For this review, take the finished solid that the model builds, in its own axes (mm). A direction names the side the tool comes from. Coordinates: 2 decimals unless noted, no trailing zeros. Loops run counter-clockwise (first coordinate to the right, second up) from the corner with the lowest first, then second, coordinate; pieces in that order, holes last. Notation, with made-up numbers: (-39.75, 5) -> (7.25, 5) arc R5 ccw to (7.25, 10) -> close; hole circle Ø3 at (79.5, -27.5). An arc over 180 degrees is marked (long way). Answer in a Markdown table with one row per item.
from build123d import *

# Parameters (mm, degrees)
BOSS_EXTRUDE1_DEPTH                           = 1
BOSS_EXTRUDE2_DEPTH                           = 1.44
CUT_EXTRUDE1_DEPTH                            = 32.926898982
SKETCH4_W                                     = 11.303
SKETCH4_H                                     = 6.1214
CUT_EXTRUDE2_DEPTH                            = 0.551
CUT_EXTRUDE2_DRAFT                            = -45
SKETCH5_R                                     = 1.7907
BOSS_EXTRUDE3_DEPTH                           = 3.8354
CSK_FOR_4_FLAT_HEAD_MACHINE_SCREW1_AT_2_COUNT = 2
CSK_FOR_4_FLAT_HEAD_MACHINE_SCREW1_AT_2_PITCH = 13.97
CUT_EXTRUDE3_START                            = -0.508
CUT_EXTRUDE3_DEPTH                            = 31.455448587
CUT_EXTRUDE3_OTHER_WAY_DEPTH                  = 2.6924
CUT_EXTRUDE3_OTHER_WAY_TAPER                  = 45
CHAMFER1_SIZE                                 = 0.762


with BuildPart() as part:
    # Sketch1 → Boss-Extrude1 (new body)
    with BuildSketch(Plane.XY):
        Polygon((-23.54, 16.9654), (-6.35, 16.9654), (6.35, 16.9654), (23.54, 16.9654), (23.54, 0), (-23.54, 0), align=None)
    extrude(amount=-BOSS_EXTRUDE1_DEPTH)

    # Sketch2 → Boss-Extrude2 (add)
    with BuildSketch(Plane.XZ):
        with BuildLine():
            Line((-23.54, 0), (-23.54, -1))
            Line((-23.54, -1), (23.54, -1))
            Line((23.54, -1), (23.54, 0))
            Line((23.54, 0), (23.54, 7.434399914))
            ThreePointArc((23.54, 7.434399914), (22.424076836, 10.12847675), (19.73, 11.244399914))
            Line((19.73, 11.244399914), (-19.73, 11.244399914))
            ThreePointArc((-19.73, 11.244399914), (-22.424076836, 10.12847675), (-23.54, 7.434399914))
            Line((-23.54, 7.434399914), (-23.54, 0))
        make_face()
    extrude(amount=BOSS_EXTRUDE2_DEPTH)

    # Sketch3 → Cut-Extrude1 (cut, through all)
    with BuildSketch(Plane.XZ.offset(1.44)):
        Polygon((4.1275, 1.143), (4.1275, 3.035802139), (2.946902139, 4.2164), (-2.946902139, 4.2164), (-4.1275, 3.035802139), (-4.1275, 1.143), align=None)
    extrude(amount=-CUT_EXTRUDE1_DEPTH, mode=Mode.SUBTRACT)


with BuildPart() as cut_extrude2_tool:
    # Sketch4 → Cut-Extrude2 (with draft: the straight prism first)
    with BuildSketch(Plane.XZ.offset(1.44)):
        with Locations((0, 2.6797)):
            Rectangle(SKETCH4_W, SKETCH4_H)
    extrude(amount=-CUT_EXTRUDE2_DEPTH)
    # Cut-Extrude2: the draft: its side faces are tilted about the plane it starts from
    cut_extrude2_sides = [cut_extrude2_tool.faces().sort_by_distance(p)[0] for p in [
        (5.6515, -1.1645, 2.6797),
        (0, -1.1645, 5.7404),
        (-5.6515, -1.1645, 2.6797),
        (0, -1.1645, -0.381),
    ]]
    draft(cut_extrude2_sides, Plane.XZ.offset(1.44), CUT_EXTRUDE2_DRAFT)


with BuildPart() as part_1:
    add(part.part)

    # Cut-Extrude2: cut by cut_extrude2_tool
    add(cut_extrude2_tool.part, mode=Mode.SUBTRACT)

    # Sketch5 → Boss-Extrude3 (add)
    # profile 1 of 2: a face of its own
    with BuildSketch(Plane.XY):
        with BuildLine():
            Line((10.2157, 0), (10.2157, 2.3368))
            ThreePointArc((10.2157, 2.3368), (6.985, 5.5675), (3.7543, 2.3368))
            Line((3.7543, 2.3368), (3.7543, 0))
            Line((3.7543, 0), (10.2157, 0))
        make_face()
        with Locations(Location((6.985, 2.3368, 0), (0, 0, 90))):
            Circle(SKETCH5_R, mode=Mode.SUBTRACT)
    # profile 2 of 2: a face of its own
    with BuildSketch(Plane.XY):
        with BuildLine():
            Line((-3.7543, 0), (-3.7543, 2.3368))
            ThreePointArc((-3.7543, 2.3368), (-6.985, 5.5675), (-10.2157, 2.3368))
            Line((-10.2157, 2.3368), (-10.2157, 0))
            Line((-10.2157, 0), (-3.7543, 0))
        make_face()
        with Locations(Location((-6.985, 2.3368, 0), (0, 0, 90))):
            Circle(SKETCH5_R, mode=Mode.SUBTRACT)
    extrude(amount=BOSS_EXTRUDE3_DEPTH)

    # Sketch7 → CSK for #4 Flat Head Machine Screw1 (revolve, cut)
    with BuildSketch(Plane(origin=(6.985, 2.3368, -1), x_dir=(0, 1, 0), z_dir=(1, 0, 0))):
        Polygon((0, 0), (0, 12.244399914), (1.63195, 12.244399914), (1.63195, 1.663834001), (2.8575, 0.254), (2.8575, 0), align=None)
    csk_for_4_flat_head_machine_screw1 = revolve(axis=Axis((6.985, 2.3368, -7.35), (0, 0, 1)), mode=Mode.SUBTRACT)

    # CSK for #4 Flat Head Machine Screw1 at 2: CSK for #4 Flat Head Machine Screw1 ×2
    with Locations(*[(-i * CSK_FOR_4_FLAT_HEAD_MACHINE_SCREW1_AT_2_PITCH, 0, 0) for i in range(1, CSK_FOR_4_FLAT_HEAD_MACHINE_SCREW1_AT_2_COUNT)]):
        add(csk_for_4_flat_head_machine_screw1, mode=Mode.SUBTRACT)

    # Sketch8 → Cut-Extrude3 (cut)
    with BuildSketch(Plane.XY.offset(3.8354).offset(CUT_EXTRUDE3_START)):
        Polygon((-4.6355, 0), (4.6355, 0), (4.6355, 4.535000865), (11.25247277, 4.535000865), (11.25247277, 13.015959744), (-11.892824973, 13.015959744), (-11.892824973, 4.635051274), (-4.6355, 4.635051274), align=None)
    extrude(amount=CUT_EXTRUDE3_DEPTH, mode=Mode.SUBTRACT)

    # Sketch8 → Cut-Extrude3 other way (cut)
    with BuildSketch(Plane.XY.offset(3.8354).offset(CUT_EXTRUDE3_START)):
        Polygon((-4.6355, 0), (4.6355, 0), (4.6355, 4.535000865), (11.25247277, 4.535000865), (11.25247277, 13.015959744), (-11.892824973, 13.015959744), (-11.892824973, 4.635051274), (-4.6355, 4.635051274), align=None)
    extrude(amount=-CUT_EXTRUDE3_OTHER_WAY_DEPTH, taper=CUT_EXTRUDE3_OTHER_WAY_TAPER, mode=Mode.SUBTRACT)

    # Chamfer1
    # the kernel refuses this chamfer: 0.762 mm, written as the material it takes off along each edge
    with BuildSketch(Plane(origin=(-25.499622437, -1.44, -1), x_dir=(0, 0.9996219169112966, -0.027495876610586417), z_dir=(1, 0, 0))) as chamfer1_piece_1:
        Polygon((CHAMFER1_SIZE * 0.999621916911, CHAMFER1_SIZE * 0.0274958766106), (-CHAMFER1_SIZE * 0.0274958766106, CHAMFER1_SIZE * 0.999621916911), (0, 0), align=None)
    extrude(amount=50.999244874, mode=Mode.SUBTRACT)


solid = part_1.part
Item 1: Insertion check: pin 1 (1.5 mm diameter, centred on x = 1.5, z = 2, fed in from -Y); pin 2 (6.5 mm diameter, centred on x = -6.98, y = 2.34, fed in from -Z); pin 3 (1 mm diameter, centred on x = 16.5, y = 13.5, fed in from +Z); pin 4 (4 mm diameter, centred on x = 6.98, y = 2.34, fed in from -Z). Each pin has a flat end and moves straight along its axis. Give the tip position at first contact, or say it passes through.
Worked answers:
| item | result |
|---|---|
| pin 1 | through |
| pin 2 | z = -1 |
| pin 3 | z = 0 |
| pin 4 | z = 0.23 |
Item 2: Take a section at A-A, the plane x = 1.5. State the section outline as (y, z) points, and give its area (3 significant figures).
Worked answers:
| item | result |
|---|---|
| outline | (-1.44, 5.74) -> (-0.89, 5.19) -> (-0.89, 4.22) -> (0, 4.22) -> (0, 11.24) -> (-1.44, 11.24) -> close; (-1.37, -0.31) -> (-0.68, -1) -> (16.97, -1) -> (16.97, 0) -> (0, 0) -> (0, 1.14) -> (-0.89, 1.14) -> (-0.89, 0.17) -> close |
| area | 28.5 mm² |
Item 3: Take a section at B-B, the plane x = 15. State the section outline as (y, z) points, and give its area (3 significant figures).
Worked answers:
| item | result |
|---|---|
| outline | (-1.44, -0.24) -> (-0.68, -1) -> (16.97, -1) -> (16.97, 0) -> (0, 0) -> (0, 11.24) -> (-1.44, 11.24) -> close |
| area | 34.3 mm² |
Item 4: Take a section at C-C, the plane y = 1.75. Count the separate pieces of the cut face and the enclosed holes in it, and give its area (3 significant figures).
Worked answers:
| item | result |
|---|---|
| separate pieces | 3 |
| enclosed holes | 0 |
| area | 58.4 mm² |
Item 5: For L1, parallel to Z at x = 21.5, y = 1; L2, parallel to Y at x = 0, z = 9.25; L3, parallel to X at y = 1.75, z = 3, list the stretches that pass through material, from the lowest coordinate up.
Worked answers:
| item | result |
|---|---|
| L1 | -1 to 0 |
| L2 | -1.44 to 0 |
| L3 | -10.22 to -8.68, -5.29 to -4.31, 4.31 to 5.29, 8.68 to 10.22 |
Item 6: Take a section at D-D, the plane z = 6.5. State the section outline as (x, y) points.
Worked answers:
| item | result |
|---|---|
| outline | (-23.54, -1.44) -> (23.54, -1.44) -> (23.54, 0) -> (-23.54, 0) -> close |
Item 7: The part is to be moulded in two halves that separate along X. For faces 1 (the cylindrical face through (22.45, -0.71, 10.1)), 2 (the flat face through (0, 8, -1)), 3 (the flat face through (-0.1, 0, 0.6)), say which applies: +X half, -X half, draft (parallel to the pull), parting line (faces both ways), or undercut.
Worked answers:
| item | result |
|---|---|
| face 1 | +X half |
| face 2 | draft |
| face 3 | undercut |
Item 8: For faces 4 (the flat face through (-10.216, 1, 2)), 5 (the flat face through (0, -0.5, 4.216)), 6 (the flat face through (-4.128, -0.5, 2.1)), 7 (the cylindrical face through (7.056, 5.567, 1.465)), list the 3-axis set-ups (+Z, -Z, +X, -X, +Y, -Y) from which the entire face can be reached by the end or side of a thin tool; tool diameter is ignored.
Worked answers:
| item | result |
|---|---|
| face 4 | +Z, -X, +Y |
| face 5 | +Y, -Y |
| face 6 | -Y |
| face 7 | +Z, +Y |
